```python
from build123d import *

# Parameters (mm, degrees)
SKETCH1_W           = 249.6
SKETCH1_H           = 284.42
SKETCH1_R           = 2.5
SKETCH1_W_2         = 33
SKETCH1_H_2         = 90
BOSS_EXTRUDE1_DEPTH = 5
SKETCH4_W           = 135
SKETCH4_H           = 244.46665057
CUT_EXTRUDE2_DEPTH  = 49.034766894
CUT_EXTRUDE3_DEPTH  = 6
CUT_EXTRUDE4_DEPTH  = 6
SKETCH7_W           = 5
SKETCH7_H           = 20
SKETCH7_H_2         = 25
CUT_EXTRUDE5_DEPTH  = 6


with BuildPart() as part:
    # Sketch1 → Boss-Extrude1 (new body)
    with BuildSketch(Plane.XY):
        with Locations((124.8, -142.21)):
            Rectangle(SKETCH1_W, SKETCH1_H)
        with Locations((245.6, -26.5)):
            Circle(SKETCH1_R, mode=Mode.SUBTRACT)
        with Locations((245.6, -77.5)):
            Circle(SKETCH1_R, mode=Mode.SUBTRACT)
        with Locations((4, -77.5)):
            Circle(SKETCH1_R, mode=Mode.SUBTRACT)
        with Locations((4, -26.5)):
            Circle(SKETCH1_R, mode=Mode.SUBTRACT)
        with Locations((201.66, -52)):
            Rectangle(SKETCH1_W_2, SKETCH1_H_2, mode=Mode.SUBTRACT)
        with Locations((47.94, -52)):
            Rectangle(SKETCH1_W_2, SKETCH1_H_2, mode=Mode.SUBTRACT)
    extrude(amount=BOSS_EXTRUDE1_DEPTH)

    # Sketch4 → Cut-Extrude2 (cut, through all)
    with BuildSketch(Plane(origin=(0, -141.18753923, 110.307795042), x_dir=(1, 0, 0), z_dir=(0, 0.788010754, -0.615661475))):
        with Locations((67.5, 84.166930672)):
            Rectangle(SKETCH4_W, SKETCH4_H)
    extrude(amount=-CUT_EXTRUDE2_DEPTH, mode=Mode.SUBTRACT)

    # Sketch5 → Cut-Extrude3 (cut, through all)
    with BuildSketch(Plane.XY.offset(5)):
        Polygon((76.149175745, -159.084342324), (158.149444505, -51.841832454), (328.08312673, -181.777318211), (207.31876811, -339.716714228), (135, -284.42), (135, -200.788988557), align=None)
    extrude(amount=-CUT_EXTRUDE3_DEPTH, mode=Mode.SUBTRACT)

    # Sketch6 → Cut-Extrude4 (cut, through all)
    with BuildSketch(Plane.XY.offset(5)):
        Polygon((0, -94.564658056), (67.52306177, -146.194456905), (40.18963885, -181.941960195), (-27.33342292, -130.312161346), align=None)
    extrude(amount=-CUT_EXTRUDE4_DEPTH, mode=Mode.SUBTRACT)

    # Sketch7 → Cut-Extrude5 (cut, through all)
    with BuildSketch(Plane.XY.offset(5)):
        with Locations((17.788155616, -47.477871486)):
            Rectangle(SKETCH7_W, SKETCH7_H)
        with Locations((231.811844384, -47.477871486)):
            Rectangle(SKETCH7_W, SKETCH7_H)
        with Locations((17.788155616, -89.977871486)):
            Rectangle(SKETCH7_W, SKETCH7_H_2)
        with Locations((231.811844384, -89.977871486)):
            Rectangle(SKETCH7_W, SKETCH7_H_2)
    extrude(amount=-CUT_EXTRUDE5_DEPTH, mode=Mode.SUBTRACT)


solid = part.part
```
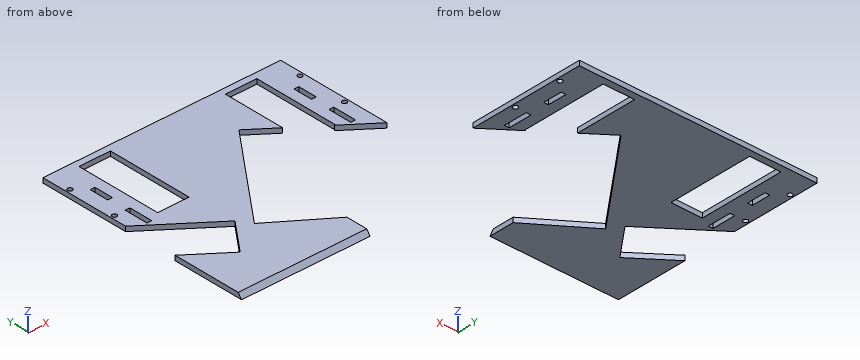
Build history of the part. All positions in model axes, mm. Round coordinates to 2 decimals unless told otherwise and drop trailing zeros. Loops run counter-clockwise (first coordinate to the right, second up) from the corner with the lowest first, then second, coordinate; pieces in that order, holes last.
Item 1: Pin check, flat tips, straight feed: P1, Ø1.5, axis at x = 231.5, z = 3, coming from the -Y side; P2, Ø1.5, axis at y = -210, z = 3.5, coming from the +X side. Stop position of each tip, or through.
Item 2: Drill centre lines: line 1 along X through (y, z) = (-44.5, 0.5); line 2 along X through (y, z) = (-29.5, 2.15); line 3 along Y through (x, z) = (4, 4.05). Where is each one in solid material? Low to high.
Item 3: Saw through at D-D (z = 1.8). State how many separate pieces and enclosed holes the cut face has, then the cut area to 3 significant figures.
Item 4: Saw through at A-A (x = 94.5). List the corners of the cut face in (y, z), then the cut area to 3 significant figures.
Item 5: Saw through at C-C (x = 202). List the corners of the cut face in (y, z), then the cut area to 3 significant figures.
Item 6: Saw through at B-B (y = -162.5). List the corners of the cut face in (x, z).
Worked answers:
1. P1: stops at y = -108.5
1. P2: stops at x = 135
2. line 1: x = 0 to 15.29, 20.29 to 31.44, 64.44 to 185.16, 218.16 to 229.31, 234.31 to 249.6
2. line 2: x = 0 to 31.44, 64.44 to 185.16, 218.16 to 249.6
2. line 3: y = -224.21 to -154.27, -97.62 to -80, -75 to -29, -24 to 0
3. separate pieces: 1
3. enclosed holes: 9
3. area: 27,400 mm2
4. outline: (-227.37, 0) - (-172.09, 0) - (-172.09, 5) - (-223.46, 5) - close; (-135.08, 0) - (0, 0) - (0, 5) - (-135.08, 5) - close
4. area: 942 mm2
5. outline: (-7, 0) - (0, 0) - (0, 5) - (-7, 5) - close
5. area: 35.0 mm2
6. outline: (0, 0) - (14.76, 0) - (14.76, 5) - (0, 5) - close; (55.06, 0) - (80.97, 0) - (80.97, 5) - (55.06, 5) - close
